from build123d import *

# Parameters (mm, degrees)
F1_W     = 60
F1_H     = 120
F1_W_2   = 55
F1_H_2   = 115
F1_W_3   = 50
F1_H_3   = 110
F2_DEPTH = 20
F3_W     = 55
F3_H     = 115
F5_DEPTH = 10
F0_W     = 60
F0_H     = 120
F6_DEPTH = 5
F7_R     = 5


with BuildPart() as f2:
    # F1 (on face) → F2 (new body)
    with BuildSketch(Plane.XZ):
        with Locations((6.1764717102, 26.1096255195)):
            Rectangle(F1_W, F1_H)
        with Locations((6.14081949, 26.4180475473)):
            Rectangle(F1_W_2, F1_H_2, mode=Mode.SUBTRACT)
        with Locations((6.14081949, 26.4180475473)):
            Rectangle(F1_W_2, F1_H_2)
        with Locations((6.5019752085, 26.4363238215)):
            Rectangle(F1_W_3, F1_H_3, mode=Mode.SUBTRACT)
    extrude(amount=F2_DEPTH)

    # F3 (on face) → F5 (join)
    with BuildSketch(Plane.XZ.offset(20)):
        Polygon((36.1764717102, 86.1096255195), (-23.8235282898, 86.1096255195), (-23.8235282898, 83.6096255195), (-23.8235282898, -33.8903744805), (36.1764717102, -33.8903744805), align=None)
        with Locations((6.1764717102, 26.1096255195)):
            Rectangle(F3_W, F3_H, mode=Mode.SUBTRACT)
    extrude(amount=F5_DEPTH)

    # F0 (on Front) → F6 (join)
    with BuildSketch(Plane.XZ):
        with Locations((6.1764717102, 26.1096255195)):
            Rectangle(F0_W, F0_H)
    extrude(amount=F6_DEPTH)

    # F7
    f7_edges = [f2.edges().sort_by_distance(p)[0] for p in [
        (36.176472, -15, 86.109626),
        (36.176472, 0, 26.109626),
        (6.176472, 0, 86.109626),
        (-23.823528, -15, 86.109626),
        (-23.823528, 0, 26.109626),
        (6.176472, 0, -33.890374),
        (36.176472, -15, -33.890374),
        (-23.823528, -15, -33.890374),
    ]]
    fillet(f7_edges, radius=F7_R)


solid = f2.part
Read the model definition and answer for the solid it produces. Units are mm, in the model's axes. A direction names the side the tool comes from. Give positions to 0.01 mm unless a question says otherwise; leave off trailing zeros. Write each loop counter-clockwise with the first axis right and the second up, starting at its lowest first coordinate (ties: lowest second). Pieces come first, ordered by that corner, then holes. Notation, with made-up numbers: (39, 43.5) - (79, 43.5) arc R14 ccw to (79, 59.5) - close; hole circle Ø9 at (43.5, 45). An arc over 180 degrees is marked (long way). Use CSV: the item, a comma, the result in double quotes. Start each with the question number.
Item 1: The part is cut by section B-B, the plane x = 11. Give the vertices of the cut face in (y, z), and give its area (3 significant figures).
Item 2: The mould has two halves that part along X. Classify faces 1 (the flat face through (-20, -20, 26)), 2 (the cylindrical face through (34.673, -17.325, -32.465)), 3 (the flat face through (-23.824, -17, 27)): pulls with the +X half, pulls with the -X half, needs draft (parallel to the pull), parting line crosses it, or undercut.
Item 3: For faces 4 (the flat face through (33.676, -25, 25)), 5 (the cylindrical face through (6.53, -1.43, -32.39)), determine the directions among +Z, -Z, +X, -X, +Y, -Y from which every point of the face is accessible in a straight line to the end or side of a thin tool.
Item 4: The part is cut by section C-C, the plane z = 4. Give the vertices of the cut face in (x, y), and give its area (3 significant figures).
Item 5: The part is cut by section A-A, the plane y = -14.5. Give the vertices of the cut face in (x, z).
Item 6: A flat-ended cylindrical pin translates along its axis: P1, Ø6, axis at x = 14.5, z = 2, coming from the -Y side. Find the tip coordinate at first contact, or state that the pin passes through.
Item 7: Consider line 1 (Z direction, x = 30, y = -13.25); line 2 (X direction, y = -13.75, z = -22); line 3 (X direction, y = -21.25, z = 40.5). Determine where each line is inside the solid, lowest interval first.
Item 8: The part is cut by section D-D, the plane y = -22.25. Give the vertices of the cut face in (x, z), and give its area (3 significant figures).
Taken from the geometry:
1,outline,"(-30, -33.89) - (-5, -33.89) arc R5 ccw to (0, -28.89) - (0, 81.11) arc R5 ccw to (-5, 86.11) - (-30, 86.11) - (-30, 83.61) - (-20, 83.61) - (-20, 81.44) - (-5, 81.44) - (-5, -28.56) - (-20, -28.56) - (-20, -31.39) - (-30, -31.39) - close"
1,area,"789 mm2"
2,face 1,"undercut"
2,face 2,"pulls with the +X half"
2,face 3,"pulls with the -X half"
3,face 4,"-Y"
3,face 5,"-Z, +X, -X, +Y"
4,outline,"(-23.82, -30) - (-21.32, -30) - (-21.32, -20) - (-18.5, -20) - (-18.5, -5) - (31.5, -5) - (31.5, -20) - (33.68, -20) - (33.68, -30) - (36.18, -30) - (36.18, -5) arc R5 ccw to (31.18, 0) - (-18.82, 0) arc R5 ccw to (-23.82, -5) - close"
4,area,"489 mm2"
5,outline,"(-23.82, -28.89) arc R5 ccw to (-18.82, -33.89) - (31.18, -33.89) arc R5 ccw to (36.18, -28.89) - (36.18, 81.11) arc R5 ccw to (31.18, 86.11) - (-18.82, 86.11) arc R5 ccw to (-23.82, 81.11) - close; hole (-18.5, -28.56) - (31.5, -28.56) - (31.5, 81.44) - (-18.5, 81.44) - close"
6,P1,"y = -5"
7,line 1,"-33.89 to -28.56, 81.44 to 86.11"
7,line 2,"-23.82 to -18.5, 31.5 to 36.18"
7,line 3,"-23.82 to -21.32, 33.68 to 36.18"
8,outline,"(-23.82, -28.89) arc R5 ccw to (-18.82, -33.89) - (31.18, -33.89) arc R5 ccw to (36.18, -28.89) - (36.18, 81.11) arc R5 ccw to (31.18, 86.11) - (-18.82, 86.11) arc R5 ccw to (-23.82, 81.11) - close; hole (-21.32, -31.39) - (33.68, -31.39) - (33.68, 83.61) - (-21.32, 83.61) - close"
8,area,"854 mm2"
